Build history of the part. All positions in model axes, mm. Face numbers are marked on the shaded views. A direction names the side the tool comes from. Give positions to 0.01 mm unless a question says otherwise; leave off trailing zeros. Order: outer loops, then holes, each group sorted by start corner. A loop starts at its lowest first (then second) coordinate and runs counter-clockwise, first axis right, second up. Notation, with made-up numbers: (16, -0.75) - (23, -0.75) arc R17 ccw to (23, 18.25) - close; hole circle Ø2 at (-7.5, 14). An arc over 180 degrees is marked (long way). Answer in a Markdown table with one row per item.
```python
from build123d import *

# Parameters (mm, degrees)
SKETCH1_R                = 8
SKETCH1_R_2              = 4
BOSS_EXTRUDE1_DEPTH      = 10
SKETCH2_W                = 40
SKETCH2_H                = 10
BOSS_EXTRUDE3_DEPTH      = 2
BOSS_EXTRUDE3_DEPTH_BACK = 2
FILLET1_R                = 3


with BuildPart() as part:
    # Sketch1 → Boss-Extrude1 (new body)
    with BuildSketch(Plane.XY):
        Circle(SKETCH1_R)
        Circle(SKETCH1_R_2, mode=Mode.SUBTRACT)
    extrude(amount=-BOSS_EXTRUDE1_DEPTH)

    # Sketch2 → Boss-Extrude3 (add, two sides)
    with BuildSketch(Plane(origin=(0, -8, 0), x_dir=(-1, 0, 0), z_dir=(0, -1, 0))) as boss_extrude3_sk:
        with Locations((0, 5)):
            Rectangle(SKETCH2_W, SKETCH2_H)
    extrude(amount=BOSS_EXTRUDE3_DEPTH)
    extrude(boss_extrude3_sk.sketch, amount=-BOSS_EXTRUDE3_DEPTH_BACK)

    # Fillet1
    fillet1_edges = [part.edges().sort_by_distance(p)[0] for p in [
        (5.291502622, -6, -5),
        (-5.291502622, -6, -5),
    ]]
    fillet(fillet1_edges, radius=FILLET1_R)


solid = part.part
```
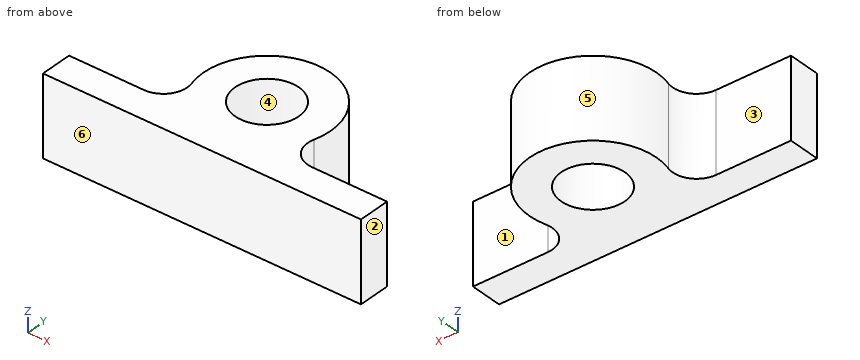
1. Cut at A-A on y = 0. Write the cut outline in (x, z).
Check result:
| item | result |
|---|---|
| outline | (-8, -10) - (-4, -10) - (-4, 0) - (-8, 0) - close; (4, -10) - (8, -10) - (8, 0) - (4, 0) - close |
2. Drop flat-ended pins along their axis: P1, Ø4, axis at y = 4.5, z = -7.5, coming from the +X side; P2, Ø4.5, axis at x = -17, z = -3, coming from the +Y side; P3, Ø2, axis at x = -2, z = -5.5, coming from the +Y side; P4, Ø5, axis at x = 0, y = 0, coming from the +Z side. Give the stop position or say it passes through.
Check result:
| item | result |
|---|---|
| P1 | stops at x = 7.6 |
| P2 | stops at y = -6 |
| P3 | stops at y = 7.94 |
| P4 | passes through |
3. Cut at D-D on x = 17. Write the cut outline in (y, z), and give its area (3 significant figures).
Check result:
| item | result |
|---|---|
| outline | (-10, -10) - (-6, -10) - (-6, 0) - (-10, 0) - close |
| area | 40.0 mm² |
4. Probe line 1 (Y direction, x = 0, z = -6); line 2 (Y direction, x = -3, z = -4); line 3 (Y direction, x = 11, z = -8.25). List the from-to ranges inside material, lowest first.
Check result:
| item | result |
|---|---|
| line 1 | y = -10 to -4, 4 to 8 |
| line 2 | y = -10 to -2.65, 2.65 to 7.42 |
| line 3 | y = -10 to -6 |
5. Cut at C-C on z = -7.25. Write the cut outline in (x, y).
Check result:
| item | result |
|---|---|
| outline | (-20, -10) - (20, -10) - (20, -6) - (10.58, -6) arc R3 cw to (7.7, -2.18) arc R8 ccw (long way) to (-7.7, -2.18) arc R3 cw to (-10.58, -6) - (-20, -6) - close; hole circle Ø8 at (0, 0) |
6. Which spindle directions (+Z, -Z, +X, -X, +Y, -Y) get a long thin tool onto all of the face, cutting with end or side? Do the marked faces 1, 2 and 3. Say none if no direction does.
Check result:
| item | result |
|---|---|
| face 1 | +Z, -Z, +X, +Y |
| face 2 | +Z, -Z, +X, +Y, -Y |
| face 3 | +Z, -Z, -X, +Y |
7. Cut at B-B on x = 0. Write the cut outline in (y, z), and give its area (3 significant figures).
Check result:
| item | result |
|---|---|
| outline | (-10, -10) - (-4, -10) - (-4, 0) - (-10, 0) - close; (4, -10) - (8, -10) - (8, 0) - (4, 0) - close |
| area | 100 mm² |
8. Two-plate mould, pull along X, no slides. Class the marked faces 4, 5 and 6: +X half, -X half, draft (parallel to the pull), parting line (faces both ways), or undercut.
Check result:
| item | result |
|---|---|
| face 4 | undercut |
| face 5 | parting line |
| face 6 | draft |
